from build123d import *

# Parameters (mm, degrees)
F1_FACE1_R = 25.6771243445
F3_DEPTH   = 8
F4_R       = 5
F5_DEPTH   = 3


with BuildPart() as f1:
    # F0 (on Front) → F1 (revolve)
    with BuildSketch(Plane.XZ):
        with BuildLine():
            Line((0, 25.6771243445), (0, 0))
            Line((0, 0), (3, 0))
            Line((3, 0), (8, 0))
            Line((8, 0), (8, 5))
            Line((8, 5), (4, 5))
            ThreePointArc((4, 5), (3.2928932188, 5.2928932188), (3, 6))
            Line((3, 6), (3, 25.6771243445))
            ThreePointArc((3, 25.6771243445), (1.5, 25), (0, 25.6771243445))
        make_face()
    revolve(axis=Axis((1.5, 0, 0), (-1, 0, 0)))

    # F2 (on face) + F1_face1 (on face) → F3 (cut)
    with BuildSketch(Plane.YZ.offset(8)):
        with BuildLine():
            Line((-1.8, 2.0124611797), (-1.8, -2.0124611797))
            ThreePointArc((-1.8, -2.0124611797), (0, -2.7), (1.8, -2.0124611797))
            Line((1.8, -2.0124611797), (1.8, 2.0124611797))
            ThreePointArc((1.8, 2.0124611797), (0, 2.7), (-1.8, 2.0124611797))
        make_face()
    with BuildSketch(Plane(origin=(0, 0, 0), x_dir=(0, -1, 0), z_dir=(-1, 0, 0))):
        Circle(F1_FACE1_R)
    extrude(amount=-F3_DEPTH, dir=(1, 0, 0), mode=Mode.SUBTRACT)

    # F4 (on face) → F5 (cut, through all)
    with BuildSketch(Plane(origin=(0, 0, 0), x_dir=(0, -1, 0), z_dir=(-1, 0, 0))):
        with Locations((0, 12.5)):
            Circle(F4_R)
        with Locations((10.8253175473, 6.25)):
            Circle(F4_R)
        with Locations((10.8253175473, -6.25)):
            Circle(F4_R)
        with Locations((0, -12.5)):
            Circle(F4_R)
        with Locations((-10.8253175473, -6.25)):
            Circle(F4_R)
        with Locations((-10.8253175473, 6.25)):
            Circle(F4_R)
    extrude(amount=-F5_DEPTH, mode=Mode.SUBTRACT)


solid = f1.part
Here's how the part is built. I have some questions about the finished solid (model axes, mm). A direction names the side the tool comes from. Round coordinates to 2 decimals unless told otherwise and drop trailing zeros. Order: outer loops, then holes, each group sorted by start corner. A loop starts at its lowest first (then second) coordinate and runs counter-clockwise, first axis right, second up. Notation, with made-up numbers: M -39.5,-38.75 L -19.5,-38.75 A13 ccw -19.5,-34.75 Z; hole C 39,7.25 d11. An arc over 180 degrees is marked long. Return JSON: item names as keys, results as strings. Group by question number.
1. If we section it at A-A on y = 0: List the corners of the cut face in (x, z) for me, then the cut area to 3 significant figures.
2. If we section it at C-C on x = 5.5: List the corners of the cut face in (y, z) for me, then the cut area to 3 significant figures.
3. If we section it at B-B on z = 0: List the corners of the cut face in (x, y) for me, then the cut area to 3 significant figures.
4. If we section it at D-D on y = -10: State how many separate pieces and enclosed holes the cut face has, then the cut area to 3 significant figures.
5. If we mould it in two halves opening along Y, with no side actions, what happens to faces 1 (the face through (5.97, -4.88, -1.08)), 2 (the face through (1.479, -2.688, -8.284)), 3 (the face through (1.48, -15.44, -8.17)), 4 (the face through (8, -2, 0))? For each: pulls with the +Y half, pulls with the -Y half, needs draft (parallel to the pull), parting line crosses it, or undercut.
6. I'm going to push flat-ended pins straight in: pin 1 Ø5 at (y, z) = (-19, 18.5) entering from +X; pin 2 Ø3 at (x, z) = (4, -0.5) entering from -Y; pin 3 Ø1.5 at (x, z) = (5, 6.5) entering from -Y. Where does each tip first touch, or does it pass through?
7. Please list where these lines run through material, in increasing order: probe 1 along Z at (x, y) = (1.25, 1.5) (3 decimals); probe 2 along Z at (x, y) = (1.75, -7); probe 3 along X at (y, z) = (8, 17.5).
8. On a 3-axis mill with a long thin cutter (end or side, diameter ignored), from which of +Z, -Z, +X, -X, +Y, -Y can I reach the whole of each face in a straight line? I mean faces 5 (the face through (0, -5, 0)), 6 (the face through (4, -1.8, 0)). Say none if no direction works.
Reply:
{
 "1": {"outline": "M 0,-25.68 A2 cw 3,-25.68 L 3,-17.5 L 0,-17.5 Z; M 0,-7.5 L 3,-7.5 L 3,-6 A1 cw 4,-5 L 8,-5 L 8,-2.7 L 0,-2.7 Z; M 0,2.7 L 8,2.7 L 8,5 L 4,5 A1 cw 3,6 L 3,7.5 L 0,7.5 Z; M 0,17.5 L 3,17.5 L 3,25.68 A2 cw 0,25.68 Z", "area": "98.5 mm^2"},
 "2": {"outline": "C 0,0 d10; hole M -1.8,-2.01 A2.7 ccw 1.8,-2.01 L 1.8,2.01 A2.7 ccw -1.8,2.01 Z", "area": "60.7 mm^2"},
 "3": {"outline": "M 0,-25.68 A2 cw 3,-25.68 L 3,-6 A1 cw 4,-5 L 8,-5 L 8,-1.8 L 0,-1.8 Z; M 0,1.8 L 8,1.8 L 8,5 L 4,5 A1 cw 3,6 L 3,25.68 A2 cw 0,25.68 Z", "area": "173 mm^2"},
 "4": {"separate pieces": "3", "enclosed holes": "0", "area": "79.7 mm^2"},
 "5": {"face 1": "parting line crosses it", "face 2": "undercut", "face 3": "undercut", "face 4": "needs draft"},
 "6": {"pin 1": "x = 3", "pin 2": "y = -25.68", "pin 3": "through"},
 "7": {"probe 1": "-24.971 to -17.27, -7.73 to -2.245, 2.245 to 7.73, 17.27 to 24.971", "probe 2": "-24.02 to -9.47, -3.03 to 3.03, 9.47 to 24.02", "probe 3": "0 to 3"},
 "8": {"face 5": "+Z, -Z, -X, +Y, -Y", "face 6": "+X, -X"}
}
